Could you check a few things on this model? Use its own coordinates, in mm. A direction names the side the tool comes from. Give positions to 0.01 mm unless a question says otherwise; leave off trailing zeros. Write each loop counter-clockwise with the first axis right and the second up, starting at its lowest first coordinate (ties: lowest second). Pieces come first, ordered by that corner, then holes. Notation, with made-up numbers: (27, 5) - (41, 5) arc R22 cw to (41, 42) - close; hole circle Ø4 at (45.25, 7). An arc over 180 degrees is marked (long way). Use one line per item in the form item = value.
```python
from build123d import *

# Parameters (mm, degrees)
FILLET1_R     = 2
CHAMFER1_SIZE = 0.381


with BuildPart() as part:
    # Sketch1 → Revolve1 (revolve)
    with BuildSketch(Plane.XY, mode=Mode.PRIVATE) as revolve1_sk:
        Polygon((0, -111.618928003), (0, 111.618928003), (6, 111.618928003), (6, 101.618928003), (2.4, 101.618928003), (2.4, -101.618928003), (6, -101.618928003), (6, -111.618928003), align=None)
    revolve(revolve1_sk.sketch.rotate(Axis((0, 0, 0), (0, 1, 0)), 90), axis=Axis((0, 0, 0), (0, 1, 0)))  # turned: the seam where the file's is

    # Fillet1
    fillet1_edges = [part.edges().sort_by_distance(p)[0] for p in [
        (0, 101.618928003, 2.4),
        (0, -101.618928003, 2.4),
    ]]
    fillet(fillet1_edges, radius=FILLET1_R)

    # Chamfer1
    chamfer1_edges = [part.edges().sort_by_distance(p)[0] for p in [
        (0, -101.618928003, 6),
        (0, 101.618928003, 6),
    ]]
    chamfer(chamfer1_edges, length=CHAMFER1_SIZE)


solid = part.part
```
1. Imagine slicing it at B-B, the plane z = 0. List the corners of the cut face in (x, y) for me.
Response values:
outline = (-6, -111.62) - (6, -111.62) - (6, -102) - (5.62, -101.62) - (4.4, -101.62) arc R2 cw to (2.4, -99.62) - (2.4, 99.62) arc R2 cw to (4.4, 101.62) - (5.62, 101.62) - (6, 102) - (6, 111.62) - (-6, 111.62) - (-6, 102) - (-5.62, 101.62) - (-4.4, 101.62) arc R2 cw to (-2.4, 99.62) - (-2.4, -99.62) arc R2 cw to (-4.4, -101.62) - (-5.62, -101.62) - (-6, -102) - close
2. Imagine slicing it at A-A, the plane x = 0. List the corners of the cut face in (y, z) for me.
Response values:
outline = (-111.62, -6) - (-102, -6) - (-101.62, -5.62) - (-101.62, -4.4) arc R2 cw to (-99.62, -2.4) - (99.62, -2.4) arc R2 cw to (101.62, -4.4) - (101.62, -5.62) - (102, -6) - (111.62, -6) - (111.62, 6) - (102, 6) - (101.62, 5.62) - (101.62, 4.4) arc R2 cw to (99.62, 2.4) - (-99.62, 2.4) arc R2 cw to (-101.62, 4.4) - (-101.62, 5.62) - (-102, 6) - (-111.62, 6) - close
3. If I drill on line 1 (Y direction, x = 4, z = -2.5); line 2 (Z direction, x = 0.25, y = -73.5); line 3 (Y direction, x = 2.5, z = 1.5), over which ranges is the centre line in solid material (lowest first)? Write a range as from..to.
Response values:
line_1 = -111.62..-101.62, 101.62..111.62
line_2 = -2.39..2.39
line_3 = -111.62..-100.96, 100.96..111.62
4. Which directions (+Z, -Z, +X, -X, +Y, -Y) give clear straight access to the entire face, cutting with the end or side of a thin tool? Please do faces 4 (the face through (-2.024, -1.395, -1.29)), 5 (the face through (0, 111.619, 0)).
Response values:
face_4 = none
face_5 = +Z, -Z, +X, -X, +Y
5. If we mould it in two halves opening along Y, with no side actions, what happens to faces 1 (the face through (-1.802, 106.742, -5.723)), 2 (the face through (0, -111.619, 0)), 3 (the face through (5, -101.619, 0))? For each: pulls with the +Y half, pulls with the -Y half, needs draft (parallel to the pull), parting line crosses it, or undercut.
Response values:
face_1 = needs draft
face_2 = pulls with the -Y half
face_3 = undercut
6. For pin 1 (1 mm diameter, centred on y = -88.5, z = -0.5, fed in from +X); pin 2 (1.5 mm diameter, centred on y = -48, z = -3.5, fed in from -X); pin 3 (5 mm diameter, centred on x = -0.5, y = 40, fed in from +Z), each with a flat end and sliding along its axis, tell me the tip position at first contact or that it passes through.
Response values:
pin_1 = 2.4
pin_2 = through
pin_3 = 2.4
7. Imagine slicing it at C-C, the plane y = 19.5. List the corners of the cut face in (x, z) for me.
Response values:
outline = circle Ø4.8 at (0, 0)
